from build123d import *

# Parameters (mm, degrees)
BASPROSKE_W           = 5.5
BASPROSKE_H           = 44
TOOTHCUT_DEPTH        = 63.467991804
TEETHCUTS_COUNT       = 20
TEETHCUTS_ANGLE       = 342
BORSKE_R              = 0.5
BORE_DEPTH            = 50.0000508
CORTAR_EXTRUIR1_DEPTH = 5.5


with BuildPart() as part:
    # BasProSke → Base-Revolve (revolve)
    with BuildSketch(Plane(origin=(0, 0, 0), x_dir=(1, 0, 0), z_dir=(0, 1, 0)), mode=Mode.PRIVATE) as base_revolve_sk:
        with Locations((2.75, 22)):
            Rectangle(BASPROSKE_W, BASPROSKE_H)
    revolve(base_revolve_sk.sketch.rotate(Axis((-10, 0, 0), (1, 0, 0)), 180), axis=Axis((-10, 0, 0), (1, 0, 0)))

    # TooCutSke → ToothCut (cut, through all)
    with BuildSketch(Plane(origin=(0, 0, 0), x_dir=(0, 0, -1), z_dir=(1, 0, 0))):
        with BuildLine():
            ThreePointArc((1.961730392, 34.943978235), (0, 34.999), (-1.961730392, 34.943978235))
            ThreePointArc((-1.961730392, 34.943978235), (-3.235659864, 39.585086827), (-5.832115241, 43.637395396))
            ThreePointArc((-5.832115241, 43.637395396), (0, 44.0254), (5.832115241, 43.637395396))
            ThreePointArc((5.832115241, 43.637395396), (3.235659864, 39.585086827), (1.961730392, 34.943978235))
        make_face()
    toothcut = extrude(amount=TOOTHCUT_DEPTH, mode=Mode.SUBTRACT)

    # TeethCuts: ToothCut ×20 about axis
    teethcuts_axis = Axis((-10, 0, 0), (1, 0, 0))
    for i in range(1, TEETHCUTS_COUNT):
        add(toothcut.rotate(teethcuts_axis, i * TEETHCUTS_ANGLE / (TEETHCUTS_COUNT - 1)), mode=Mode.SUBTRACT)

    # BorSke → Bore (cut, symmetric)
    with BuildSketch(Plane(origin=(0, 0, 0), x_dir=(0, 0, -1), z_dir=(1, 0, 0))):
        with Locations(Location((0, 0, 0), (0, 0, 180))):
            Circle(BORSKE_R)
    extrude(amount=BORE_DEPTH, both=True, mode=Mode.SUBTRACT)

    # Croquis1 → Cortar-Extruir1 (cut)
    with BuildSketch(Plane(origin=(5.5, 0, 0), x_dir=(0, 0, -1), z_dir=(1, 0, 0))):
        with BuildLine():
            Line((0, 1.395), (3.615190175, 1.395))
            ThreePointArc((3.615190175, 1.395), (3.809493859, 0.709493859), (3.875, 0))
            ThreePointArc((3.875, 0), (0, -3.875), (-3.875, 0))
            ThreePointArc((-3.875, 0), (-3.809493859, 0.709493859), (-3.615190175, 1.395))
            Line((-3.615190175, 1.395), (0, 1.395))
        make_face()
    extrude(amount=-CORTAR_EXTRUIR1_DEPTH, mode=Mode.SUBTRACT)


solid = part.part
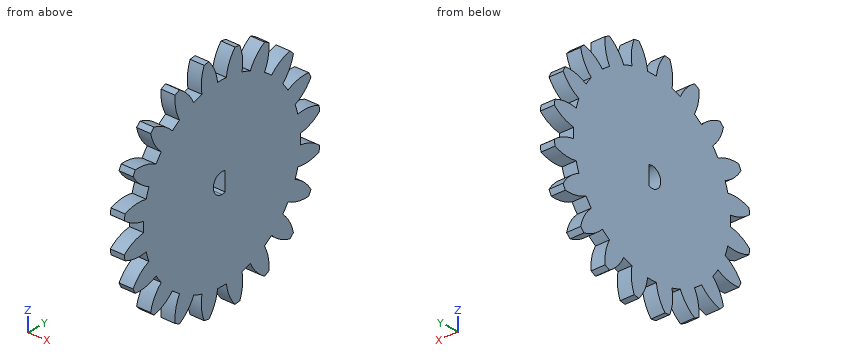
Could you check a few things on this model? Use its own coordinates, in mm. Give positions to 0.01 mm unless a question says otherwise; leave off trailing zeros. Order: outer loops, then holes, each group sorted by start corner. A loop starts at its lowest first (then second) coordinate and runs counter-clockwise, first axis right, second up. Notation, with made-up numbers: (43, -33.5) - (59, -33.5) arc R32 ccw to (59, -0.5) - close; hole circle Ø1 at (28, -11). An arc over 180 degrees is marked (long way). Return JSON: item names as keys, results as strings. Group by question number.
Q1. Suppose I cut it at B-B, the plane z = 17. Please give me the cut outline in (x, y).
Q2. Suppose I cut it at A-A, the plane z = 0. Please give me the cut outline in (x, y) (3 decimals), and give its area (3 significant figures).
Q3. Please list where these lines run through material, in increasing order: line 1 along Y through (x, z) = (0.9, -34.5); line 2 along Z through (x, y) = (0.6, 19.5); line 3 along Y through (x, z) = (3, 37.5). Write a range as [from, to].
Q4. Suppose I cut it at C-C, the plane y = 14.5. Please give me the cut outline in (x, z).
Q5. Will these pins go through, and if not, where does the flat tip stop? pin 1 Ø1 at (x, y) = (4, 21) entering from +Z; pin 2 Ø1 at (x, y) = (4.5, 8) entering from -Z; pin 3 Ø2 at (x, y) = (1.5, -12.5) entering from -Z.
Resolved:
{
 "1": {"outline": "(0, -38.27) - (5.5, -38.27) - (5.5, 38.27) - (0, 38.27) - close"},
 "2": {"outline": "(0, -34.999) - (5.5, -34.999) - (5.5, -3.875) - (0, -3.875) - close; (0, 1.395) - (5.5, 1.395) - (5.5, 34.999) - (0, 34.999) - close", "area": "356 mm2"},
 "3": {"line 1": "y = [-20.76, -13.68], [-9.05, 9.05], [13.68, 20.76]", "line 2": "z = [-39.44, -30.49], [-29.06, 29.06], [30.49, 39.44]", "line 3": "y = [-21, -16.14], [-9.23, -2.48], [2.48, 9.23], [16.14, 21]"},
 "4": {"outline": "(0, -35.67) - (5.5, -35.67) - (5.5, 35.67) - (0, 35.67) - close"},
 "5": {"pin 1": "stops at z = 38.93", "pin 2": "stops at z = -43.36", "pin 3": "stops at z = -34.21"}
}
